Print and shaded views of the part. All mm, measured from the part's lowest x, y and z. A direction names the side the tool comes from. Give positions to 0.01 mm unless a question says otherwise; leave off trailing zeros. Use one line per item in the form item = value. Start each with the question number.
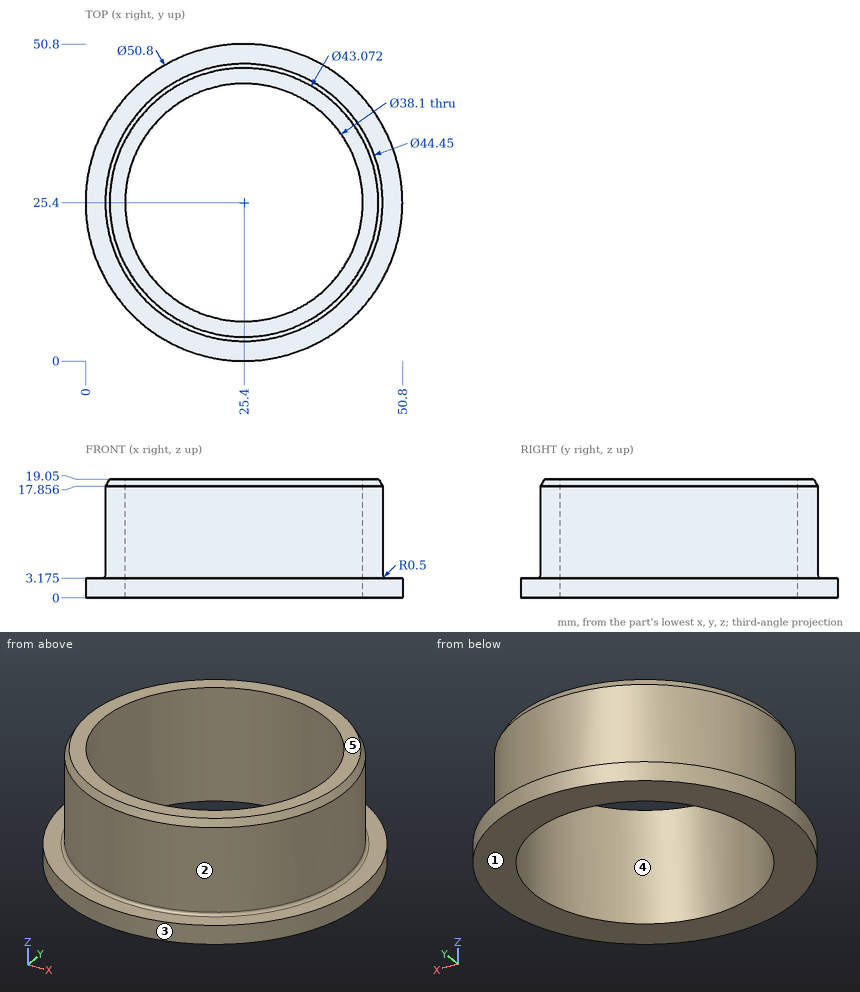
(1) Which spindle directions (+Z, -Z, +X, -X, +Y, -Y) get a long thin tool onto all of the face, cutting with end or side? Do the marked faces 1 and 2. Say none if no direction does.
(2) Wall check: line 1 (Y direction, x = 25, z = 5.25) (1 decimal); line 2 (Y direction, x = 19, z = 13.5) (1 decimal); line 3 (X direction, y = 19.5, z = 18.25) (1 decimal). Give the ranges that are in metal, low to high. Write a range as from..to.
(3) Pin check, flat tips, straight feed: pin 1 Ø4 at (x, z) = (8, 7.5) entering from -Y (1 decimal); pin 2 Ø4 at (y, z) = (16, 9.5) entering from -X; pin 3 Ø10 at (y, z) = (14.5, 7.5) entering from +X (1 decimal); pin 4 Ø4 at (x, y) = (23, 40.5) entering from -Z. Stop position of each tip, or through.
(4) Two-plate mould, pull along Y, no slides. Class the marked faces 3, 4 and 5: +Y half, -Y half, draft (parallel to the pull), parting line (faces both ways), or undercut.
Solution:
q1.face_1 = -Z, +X, -X, +Y, -Y
q1.face_2 = +Z
q2.line_1 = 3.2..6.4, 44.4..47.6
q2.line_2 = 4.1..7.5, 43.3..46.7
q2.line_3 = 4.2..7.3, 43.5..46.6
q3.pin_1 = 9.4
q3.pin_2 = 4.44
q3.pin_3 = 49.4
q3.pin_4 = through
q4.face_3 = parting line
q4.face_4 = undercut
q4.face_5 = draft
